For this review, take the finished solid that the model builds, in its own axes (mm). A direction names the side the tool comes from. Give positions to 0.01 mm unless a question says otherwise; leave off trailing zeros. Order: outer loops, then holes, each group sorted by start corner. A loop starts at its lowest first (then second) coordinate and runs counter-clockwise, first axis right, second up. Notation, with made-up numbers: M 41,78 L 83,78 A22 ccw 83,105 Z; hole C 38.25,-34 d2. An arc over 180 degrees is marked long. Answer as CSV lines item,"result". Start each with the question number.
1. We need section C-C, the plane x = 31.9. Give the boundary of the cut face in (y, z).
2. We need section B-B, the plane z = -12.5. Give the boundary of the cut face in (x, y), and give its area (3 significant figures).
3. We need section D-D, the plane y = 1.15. State how many separate pieces and enclosed holes the cut face has, and give its area (3 significant figures).
4. Machinability: for faces 4 (the flat face through (-62, 2, -30.95)), 5 (the cylindrical face through (-25.05, -1.48, 23.72)), 6 (the flat face through (-40.9, 2, -11)), which of the approach directions +Z, -Z, +X, -X, +Y, -Y give a long, thin tool a straight path to every point of the face, cutting with its end or side? Answer none if there is none.
5. Clearance check with flat-ended pins moving along their axes: P1, Ø3, axis at y = -1, z = -17, coming from the +X side; P2, Ø3, axis at x = 51.9, z = -20.95, coming from the -Y side; P3, Ø3.5, axis at y = 1, z = 8, coming from the +X side (3 decimals); P4, Ø1, axis at y = 1.5, z = 16, coming from the +X side. State where each tip first meets the part, or that it passes through.
6. Mouldability with a two-part tool opening along Z and no side actions: class faces 1 (the cylindrical face through (52.17, 1.52, 38.89)), 2 (the cylindrical face through (-61.05, 1.52, -37.94)), 3 (the flat face through (-34.549, 2, 8)) as pulls with the +Z half, pulls with the -Z half, needs draft (parallel to the pull), parting line crosses it, or undercut.
7. For line 1 along X through (y, z) = (-1.55, -30.95); line 2 along X through (y, z) = (2.35, -20.95); line 3 along X through (y, z) = (2.25, -14), list the stretches that pass through material, from the lowest coordinate up.
8. We need section A-A, the plane x = -23.9. Give the boundary of the cut face in (y, z).
from build123d import *

# Parameters (mm, degrees)
SKETCH1_R           = 3
BOSS_EXTRUDE1_DEPTH = 3
SKETCH1_3_R         = 3
BOSS_EXTRUDE2_DEPTH = 3
SKETCH3_R           = 1.75
CUT_EXTRUDE1_DEPTH  = 77.132204093
FILLET1_R           = 10
SKETCH4_R           = 1.75
CUT_EXTRUDE2_DEPTH  = 77.132204093
SKETCH5_W           = 1.5
SKETCH5_H           = 6.5
CUT_EXTRUDE3_DEPTH  = 77.132204093
LPATTERN1_COUNT     = 2
LPATTERN1_PITCH     = 20
SKETCH6_W           = 3
SKETCH6_H           = 12
CUT_EXTRUDE4_DEPTH  = 77.132204093


with BuildPart() as part:
    # Sketch1 → Boss-Extrude1 (new body)
    # profile 1 of 5: a face of its own
    with BuildSketch(Plane(origin=(0, 0, 0), x_dir=(1, 0, 0), z_dir=(0, 1, 0))):
        Polygon((-63.9, -0.95), (-53.9, -40.95), (53.9, -40.95), (63.9, -0.95), (63.9, 40.95), (-63.9, 40.95), align=None)
        with Locations((-23.9, -20.95)):
            Circle(SKETCH1_R, mode=Mode.SUBTRACT)
        with Locations((23.9, -19.85)):
            Circle(SKETCH1_R, mode=Mode.SUBTRACT)
        with Locations((-19.2, 30.95)):
            Circle(SKETCH1_R, mode=Mode.SUBTRACT)
        with Locations((8.7, 30.95)):
            Circle(SKETCH1_R, mode=Mode.SUBTRACT)
    # profile 2 of 5: a face of its own
    with BuildSketch(Plane(origin=(0, 0, 0), x_dir=(1, 0, 0), z_dir=(0, 1, 0))):
        with Locations((-23.9, -20.95)):
            Circle(SKETCH1_R)
    # profile 3 of 5: a face of its own
    with BuildSketch(Plane(origin=(0, 0, 0), x_dir=(1, 0, 0), z_dir=(0, 1, 0))):
        with Locations((23.9, -19.85)):
            Circle(SKETCH1_R)
    # profile 4 of 5: a face of its own
    with BuildSketch(Plane(origin=(0, 0, 0), x_dir=(1, 0, 0), z_dir=(0, 1, 0))):
        with Locations((-19.2, 30.95)):
            Circle(SKETCH1_R)
    # profile 5 of 5: a face of its own
    with BuildSketch(Plane(origin=(0, 0, 0), x_dir=(1, 0, 0), z_dir=(0, 1, 0))):
        with Locations((8.7, 30.95)):
            Circle(SKETCH1_R)
    extrude(amount=BOSS_EXTRUDE1_DEPTH)

    # Sketch1_3 → Boss-Extrude2 (add)
    with BuildSketch(Plane(origin=(0, 0, 0), x_dir=(1, 0, 0), z_dir=(0, 1, 0))):
        with Locations(Location((-23.9, -20.95, 0), (0, 0, 270))):
            Circle(SKETCH1_3_R)
        with Locations(Location((23.9, -19.85, 0), (0, 0, 270))):
            Circle(SKETCH1_3_R)
        with Locations(Location((-19.2, 30.95, 0), (0, 0, 270))):
            Circle(SKETCH1_3_R)
        with Locations(Location((8.7, 30.95, 0), (0, 0, 270))):
            Circle(SKETCH1_3_R)
    extrude(amount=-BOSS_EXTRUDE2_DEPTH)

    # Sketch3 → Cut-Extrude1 (cut, through all)
    with BuildSketch(Plane.XZ.offset(3)):
        with Locations(Location((8.7, -30.95, 0), (0, 0, 270))):
            Circle(SKETCH3_R)
        with Locations(Location((-19.2, -30.95, 0), (0, 0, 270))):
            Circle(SKETCH3_R)
        with Locations(Location((23.9, 19.85, 0), (0, 0, 270))):
            Circle(SKETCH3_R)
        with Locations(Location((-23.9, 20.95, 0), (0, 0, 270))):
            Circle(SKETCH3_R)
    extrude(amount=-CUT_EXTRUDE1_DEPTH, mode=Mode.SUBTRACT)

    # Fillet1
    fillet1_edges = [part.edges().sort_by_distance(p)[0] for p in [
        (-53.9, 1.5, 40.95),
        (-63.9, 1.5, 0.95),
        (-63.9, 1.5, -40.95),
        (63.9, 1.5, -40.95),
        (63.9, 1.5, 0.95),
        (53.9, 1.5, 40.95),
    ]]
    fillet(fillet1_edges, radius=FILLET1_R)

    # Sketch4 → Cut-Extrude2 (cut, through all)
    with BuildSketch(Plane(origin=(0, 3, 0), x_dir=(1, 0, 0), z_dir=(0, 1, 0))):
        with Locations(Location((51.9, 20.95, 0), (0, 0, 270))):
            Circle(SKETCH4_R)
        with Locations(Location((31.9, 20.95, 0), (0, 0, 270))):
            Circle(SKETCH4_R)
        with Locations(Location((51.9, -4.05, 0), (0, 0, 270))):
            Circle(SKETCH4_R)
        with Locations(Location((31.9, -4.05, 0), (0, 0, 270))):
            Circle(SKETCH4_R)
    extrude(amount=-CUT_EXTRUDE2_DEPTH, mode=Mode.SUBTRACT)

    # Sketch5 → Cut-Extrude3 (cut, through all)
    with BuildSketch(Plane(origin=(0, 3, 0), x_dir=(1, 0, 0), z_dir=(0, 1, 0))):
        with Locations((-47.65, 10.95)):
            Rectangle(SKETCH5_W, SKETCH5_H)
        with Locations((-40.15, 10.95)):
            Rectangle(SKETCH5_W, SKETCH5_H)
    cut_extrude3 = extrude(amount=-CUT_EXTRUDE3_DEPTH, mode=Mode.SUBTRACT)

    # LPattern1: Cut-Extrude3 ×2
    with Locations(*[Vector(0.2425356250363331, 0, 0.970142500145332) * (i * LPATTERN1_PITCH) for i in range(1, LPATTERN1_COUNT)]):
        add(cut_extrude3, mode=Mode.SUBTRACT)

    # Sketch6 → Cut-Extrude4 (cut, through all)
    with BuildSketch(Plane(origin=(0, 3, 0), x_dir=(1, 0, 0), z_dir=(0, 1, 0))):
        Polygon((58.704088438, -21.733646249), (55.793660937, -21.006039374), (52.883233437, -32.647749375), (55.793660937, -33.37535625), align=None)
        with Locations((-62.4, 24.95)):
            Rectangle(SKETCH6_W, SKETCH6_H)
        Polygon((-58.704088438, -21.733646249), (-55.793660937, -21.006039374), (-52.883233437, -32.647749375), (-55.793660937, -33.37535625), align=None)
        with Locations((62.4, 24.95)):
            Rectangle(SKETCH6_W, SKETCH6_H)
    extrude(amount=-CUT_EXTRUDE4_DEPTH, mode=Mode.SUBTRACT)


solid = part.part
Result set:
1,outline,"M 0,-40.95 L 3,-40.95 L 3,-22.7 L 0,-22.7 Z; M 0,-19.2 L 3,-19.2 L 3,2.3 L 0,2.3 Z; M 0,5.8 L 3,5.8 L 3,40.95 L 0,40.95 Z"
2,outline,"M -63.9,0 L -48.4,0 L -48.4,3 L -63.9,3 Z; M -46.9,0 L -40.9,0 L -40.9,3 L -46.9,3 Z; M -39.4,0 L 63.9,0 L 63.9,3 L -39.4,3 Z"
2,area,"374 mm2"
3,separate pieces,"1"
3,enclosed holes,"12"
3,area,"9,740 mm2"
4,face 4,"-X, +Y, -Y"
4,face 5,"-Y"
4,face 6,"+Y, -Y"
5,P1,"x = 63.9"
5,P2,"through"
5,P3,"x = 62.575"
5,P4,"x = 60.26"
6,face 1,"pulls with the +Z half"
6,face 2,"pulls with the -Z half"
6,face 3,"undercut"
7,line 1,"-22.2 to -20.95, -17.45 to -16.2, 5.7 to 6.95, 10.45 to 11.7"
7,line 2,"-60.9 to 30.15, 33.65 to 50.15, 53.65 to 60.9"
7,line 3,"-63.9 to -48.4, -46.9 to -40.9, -39.4 to 63.9"
8,outline,"M -3,17.95 L 0,17.95 L 0,-40.95 L 3,-40.95 L 3,19.2 L -3,19.2 Z; M -3,22.7 L 3,22.7 L 3,40.95 L 0,40.95 L 0,23.95 L -3,23.95 Z"
